```python
from build123d import *

# Parameters (mm, degrees)
F1_DEPTH = 6.35
F3_DEPTH = 19.05


with BuildPart() as f1:
    # F0 (on Top) → F1 (new body)
    with BuildSketch(Plane.XY):
        with BuildLine():
            Line((-11.39312, 24.096514), (-24.09312, 24.096514))
            ThreePointArc((-24.09312, 24.096514), (-28.583248, 22.236642), (-30.44312, 17.746514))
            Line((-30.44312, 17.746514), (-30.44312, -14.003486))
            Line((-30.44312, -14.003486), (33.05688, -14.003486))
            Line((33.05688, -14.003486), (33.05688, 17.746514))
            ThreePointArc((33.05688, 17.746514), (31.197008, 22.236642), (26.70688, 24.096514))
            Line((26.70688, 24.096514), (14.00688, 24.096514))
            ThreePointArc((14.00688, 24.096514), (1.30688, 11.396514), (-11.39312, 24.096514))
        make_face()
    extrude(amount=F1_DEPTH)

    # F2 (on face) → F3 (join)
    with BuildSketch(Plane.XY.offset(6.35)):
        with BuildLine():
            Line((-24.09312, 5.046514), (-24.09312, -14.003486))
            Line((-24.09312, -14.003486), (-17.74312, -14.003486))
            Line((-17.74312, -14.003486), (-17.74312, -5.113486))
            Line((-17.74312, -5.113486), (20.35688, -5.113486))
            Line((20.35688, -5.113486), (20.35688, -14.003486))
            Line((20.35688, -14.003486), (26.70688, -14.003486))
            Line((26.70688, -14.003486), (26.70688, 5.046514))
            Line((26.70688, 5.046514), (20.35688, 5.046514))
            ThreePointArc((20.35688, 5.046514), (18.560829, 5.790463), (17.81688, 7.586514))
            Line((17.81688, 7.586514), (17.81688, 24.096514))
            Line((17.81688, 24.096514), (14.00688, 24.096514))
            ThreePointArc((14.00688, 24.096514), (1.30688, 11.396514), (-11.39312, 24.096514))
            Line((-11.39312, 24.096514), (-15.20312, 24.096514))
            Line((-15.20312, 24.096514), (-15.20312, 7.620516))
            ThreePointArc((-15.20312, 7.620516), (-15.202892, 7.586514), (-15.20312, 7.552512))
            ThreePointArc((-15.20312, 7.552512), (-15.958984, 5.778401), (-17.74312, 5.046514))
            Line((-17.74312, 5.046514), (-24.09312, 5.046514))
        make_face()
    extrude(amount=F3_DEPTH)


solid = f1.part
```
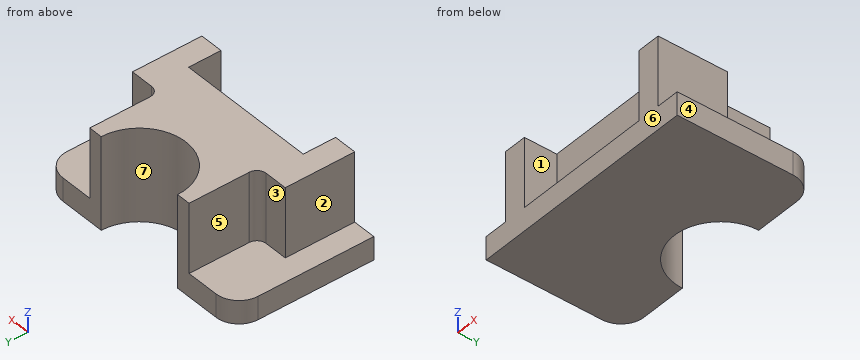
Design review of the part built by this model. Coordinates are the model's own, in mm. Face numbers are marked on the shaded views. A direction names the side the tool comes from. Round coordinates to 2 decimals unless told otherwise and drop trailing zeros. Order: outer loops, then holes, each group sorted by start corner. A loop starts at its lowest first (then second) coordinate and runs counter-clockwise, first axis right, second up. Notation, with made-up numbers: (9.5, -0.75) - (64.5, -0.75) arc R26 ccw to (64.5, 34.25) - close; hole circle Ø9 at (-23, 11). An arc over 180 degrees is marked (long way). Return JSON: item names as keys, results as strings.
Q1. Consider section A-A on y = -1.5. Write out the cut boundary in (x, z), plus the area to 3 significant figures.
Computed values:
{"outline": "(-30.44, 0) - (33.06, 0) - (33.06, 6.35) - (26.71, 6.35) - (26.71, 25.4) - (-24.09, 25.4) - (-24.09, 6.35) - (-30.44, 6.35) - close", "area": "1,370 mm2"}
Q2. Wall thickness on L1, parallel to X at y = -5.5, z = 15; L2, parallel to Y at x = -21, z = 18; L3, parallel to X at y = 17, z = 22.75: over which ranges is each line inside the solid? List them lowest first. Write a range as [from, to].
Computed values:
{"L1": "x = [-24.09, -17.74], [20.36, 26.71]", "L2": "y = [-14, 5.05]", "L3": "x = [-15.2, -9.23], [11.84, 17.82]"}
Q3. Consider section D-D on z = 21.75. Write out the cut boundary in (x, y), plus the area to 3 significant figures.
Computed values:
{"outline": "(-24.09, -14) - (-17.74, -14) - (-17.74, -5.11) - (20.36, -5.11) - (20.36, -14) - (26.71, -14) - (26.71, 5.05) - (20.36, 5.05) arc R2.54 cw to (17.82, 7.59) - (17.82, 24.1) - (14.01, 24.1) arc R12.7 cw to (-11.39, 24.1) - (-15.2, 24.1) - (-15.2, 7.62) arc R2.54 cw to (-15.2, 7.55) arc R2.54 cw to (-17.74, 5.05) - (-24.09, 5.05) - close", "area": "1,010 mm2"}
Q4. Consider section C-C on x = 22. Write out the cut boundary in (y, z), plus the area to 3 significant figures.
Computed values:
{"outline": "(-14, 0) - (24.1, 0) - (24.1, 6.35) - (5.05, 6.35) - (5.05, 25.4) - (-14, 25.4) - close", "area": "605 mm2"}
Q5. The part is to be moulded in two halves that separate along X. For the marked faces 4, 5, 6 and 7, say which applies: pulls with the +X half, pulls with the -X half, needs draft (parallel to the pull), parting line crosses it, or undercut.
Computed values:
{"face 4": "pulls with the +X half", "face 5": "pulls with the -X half", "face 6": "needs draft", "face 7": "undercut"}
Q6. For pin 1 Ø5 at (y, z) = (12.5, 18.5) entering from -X; pin 2 Ø7 at (y, z) = (-9.5, 16) entering from +X; pin 3 Ø5 at (x, z) = (-12, 19) entering from -Y; pin 4 Ø2 at (x, y) = (23.5, 13.5) entering from -Z, all flat-tipped, find the tip position at first contact; note any pin that passes through.
Computed values:
{"pin 1": "stops at x = -15.2", "pin 2": "stops at x = 26.71", "pin 3": "stops at y = -5.11", "pin 4": "stops at z = 0"}
Q7. Consider section B-B on z = 2. Write out the cut boundary in (x, y).
Computed values:
{"outline": "(-30.44, -14) - (33.06, -14) - (33.06, 17.75) arc R6.35 ccw to (26.71, 24.1) - (14.01, 24.1) arc R12.7 cw to (-11.39, 24.1) - (-24.09, 24.1) arc R6.35 ccw to (-30.44, 17.75) - close"}
Q8. Machinability: for the marked faces 1, 2 and 3, which of the approach directions +Z, -Z, +X, -X, +Y, -Y give a long, thin tool a straight path to every point of the face, cutting with its end or side? Answer none if there is none.
Computed values:
{"face 1": "+Z, -Y", "face 2": "+Z, -X, +Y, -Y", "face 3": "+Z, -X, +Y"}
